```python
from build123d import *

# Parameters (mm, degrees)
EXTRUDE_START            = -275
SKETCH_1_R               = 20
SKETCH_1_R_2             = 10
EXTRUDE_1_DEPTH          = 250
CUT_EXTRUDE_1_REACH      = 282.584
CUT_EXTRUDE_1_END_RADIUS = 10
CUT_EXTRUDE_START        = -3
SKETCH_2_W               = 250
SKETCH_2_H               = 6


with BuildPart() as part:
    # 草圖1 → 填料-伸長1 (new body)
    with BuildSketch(Plane.XY.offset(EXTRUDE_START)):
        with Locations((-0.015741253, -0.499752152)):
            Circle(SKETCH_1_R)
        Circle(SKETCH_1_R_2, mode=Mode.SUBTRACT)
    extrude(amount=EXTRUDE_1_DEPTH)

    # 除料-伸長1: up to this cylinder (the profile starts outside it)
    cut_extrude_1_end = Plane(origin=(0, 0, -150), z_dir=(0, 0, 1)) * Cylinder(CUT_EXTRUDE_1_END_RADIUS, 586.168, mode=Mode.PRIVATE)
    # 草圖2 → 除料-伸長1 (cut, up to the surface)
    with BuildSketch(Plane(origin=(-2.893904806, 9.572111312, 0), x_dir=(0, 0, 1), z_dir=(0.28939048064098244, -0.9572111312110727, 0)).offset(CUT_EXTRUDE_START), mode=Mode.PRIVATE) as cut_extrude_1_sk1:
        with Locations((-150, -0.296650626)):
            Rectangle(SKETCH_2_W, SKETCH_2_H)
    cut_extrude_1_tool1 = extrude(cut_extrude_1_sk1.sketch, amount=CUT_EXTRUDE_1_REACH, mode=Mode.PRIVATE) - cut_extrude_1_end
    add(cut_extrude_1_tool1.solids().sort_by_distance((-3.478119, 12.529593, -150))[0], mode=Mode.SUBTRACT)


solid = part.part
```
Source: CAD feature listing. Evaluate the final solid. Frame: model axes, mm. A direction names the side the tool comes from. Round coordinates to 2 decimals unless told otherwise and drop trailing zeros. Loops run counter-clockwise (first coordinate to the right, second up) from the corner with the lowest first, then second, coordinate; pieces in that order, holes last. Notation, with made-up numbers: M -34.5,-1.5 L 5.5,-1.5 A10 cw 5.5,13.5 Z; hole C -35,67.25 d11. An arc over 180 degrees is marked long. Use a Markdown table: item, result. Add a question column.
1. Line query: line 1 (X direction, y = 0, z = -217); line 2 (X direction, y = 2.5, z = -183); line 3 (Y direction, x = 9, z = -190). Output: solid intervals per line, ascending.
2. Section query A-A on y = 4.5. Return the cut outline in (x, z).
3. Reachability of faces 1 (the flat face through (-5, -9, -25)), 2 (the flat face through (-3.518, 12.517, -151.75)) from +Z, -Z, +X, -X, +Y, -Y: full face, straight path, thin tool, end or side. Return the list, or none.
4. Contact query for flat-ended pins moving along their axis: P1, Ø10, axis at y = -13, z = -79.5, coming from the -X side; P2, Ø3, axis at y = 14, z = -77.5, coming from the -X side; P3, Ø4, axis at x = 15.5, z = -78.5, coming from the -Y side. Output: stop coordinate, or through.
5. Section query C-C on x = 17. Return the cut outline in (y, z).
6. Section query D-D on y = -14.5. Return the cut outline in (x, z), then the cut area to 3 significant figures.
7. Section query B-B on z = -97. Return the cut outline in (x, y).
8. Mould query, pull axis X, two halves, no side actions, for faces 3 (the cylindrical face through (-15.887, -12.669, -151.75)), 4 (the cylindrical face through (2.209, -9.753, -151.75)), 5 (the flat face through (-5, -9, -275)). Classes: pulls with the +X half, pulls with the -X half, needs draft (parallel to the pull), parting line crosses it, or undercut.
Reported:
| question | item | result |
|---|---|---|
| 1 | line 1 | x = -20.01 to -10, 10 to 19.98 |
| 1 | line 2 | x = -19.79 to -9.68, 9.68 to 19.76 |
| 1 | line 3 | y = -18.35 to -4.36, 4.36 to 17.35 |
| 2 | outline | M -19.38,-275 L -8.93,-275 L -8.93,-25 L -19.38,-25 Z; M 8.93,-275 L 19.35,-275 L 19.35,-25 L 8.93,-25 Z |
| 3 | face 1 | +Z, +X, -X, +Y, -Y |
| 3 | face 2 | +Z, -Z |
| 4 | P1 | stops at x = -18.56 |
| 4 | P2 | stops at x = -15.21 |
| 4 | P3 | stops at y = -15.24 |
| 5 | outline | M -11.01,-275 L 10.01,-275 L 10.01,-25 L -11.01,-25 Z |
| 6 | outline | M -14.3,-275 L 14.27,-275 L 14.27,-25 L -14.3,-25 Z |
| 6 | area | 7,140 mm² |
| 7 | outline | C -0.02,-0.5 d40; hole M -6.35,11.66 L -5.37,8.43 A10 ccw long 0.42,9.99 L -0.61,13.4 Z |
| 8 | face 3 | parting line crosses it |
| 8 | face 4 | undercut |
| 8 | face 5 | needs draft |
